from build123d import *

# Parameters (mm, degrees)
SKETCH6_R = 3.175
SKETCH8_R = 3.175


with BuildPart() as part:
    # Sweep1: sweep along a path in Sketch5
    with BuildLine(Plane(origin=(0, 0, 0), x_dir=(0, 0, -1), z_dir=(1, 0, 0))) as sweep1_path:
        ThreePointArc((0, 38.1), (-8.001782337, -37.250254757), (15.646636775, 34.738922805))
    # Sketch6 → Sweep1 (sweep)
    with BuildSketch(Plane.XY):
        with Locations((0, 38.1)):
            Circle(SKETCH6_R)
    sweep(path=sweep1_path.line)

    # Sweep2: sweep along a path in Sketch7
    with BuildLine(Plane.XY) as sweep2_path:
        Line((0, 38.1), (-40.976396272, 38.1))
    # Sketch8 → Sweep2 (sweep)
    with BuildSketch(Plane(origin=(0, 0, 0), x_dir=(0, 0, -1), z_dir=(1, 0, 0))):
        with Locations((0, 38.1)):
            Circle(SKETCH8_R)
    sweep(path=sweep2_path.line)

    # Sketch9 → Revolve7 (revolve)
    with BuildSketch(Plane(origin=(0, 0, 0), x_dir=(0, 0, -1), z_dir=(1, 0, 0))):
        with BuildLine():
            Line((0, 41.275), (0, 34.925))
            ThreePointArc((0, 34.925), (3.175, 38.1), (0, 41.275))
        make_face()
    revolve(axis=Axis((0, 0, 0), (0, 1, 0)))


solid = part.part
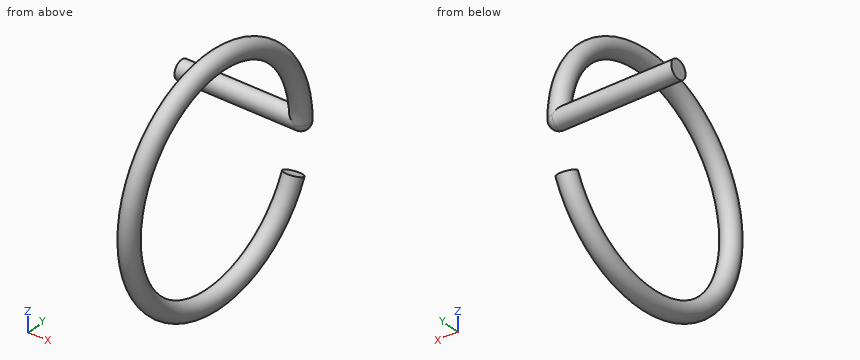
Check sheet for the modelled part. Datum: model origin and axes. Units: mm. Give positions to 0.01 mm unless a question says otherwise; leave off trailing zeros. Order: outer loops, then holes, each group sorted by start corner. A loop starts at its lowest first (then second) coordinate and runs counter-clockwise, first axis right, second up. Notation, with made-up numbers: M -7.75,24.5 L 49.25,24.5 A28 cw 49.25,60.5 Z; hole C 8.5,17.25 d1. An arc over 180 degrees is marked long. Answer as CSV lines item,"result". Start each with the question number.
Item 1: Cross-section at A-A on x = -26. Enter the section's corners in (y, z) (3 decimals), plus the area to 3 significant figures.
Item 2: Gauge pin test, flat ends, axial feed: P1, Ø4, axis at x = -3.5, y = -14, coming from the +Z side; P2, Ø1, axis at x = -5.5, y = 4, coming from the -Z side; P3, Ø8, axis at y = -26, z = 18.5, coming from the -X side; P4, Ø1.5, axis at y = -31, z = 19.5, coming from the +X side. Record the tip position at first contact, or that the pin passes through.
Item 3: Thickness scan on line 1 (Z direction, x = -26.5, y = 38); line 2 (Z direction, x = -1, y = 4); line 3 (Y direction, x = 1.5, z = 27). Record the ranges inside material, lowest first. Write a range as [from, to].
Established:
1,outline,"C 38.1,0 d6.35"
1,area,"31.7 mm^2"
2,P1,"stops at z = 38.61"
2,P2,"passes through"
2,P3,"stops at x = -2.3"
2,P4,"stops at x = 3.09"
3,line 1,"z = [-3.17, 3.17]"
3,line 2,"z = [-40.92, -34.86], [34.86, 40.92]"
3,line 3,"y = [-30.72, -22.74], [22.74, 30.72]"
